Geometry check sheet. Reference: drawing and pictorial views, mm from the part's lowest x, y, z. A direction names the side the tool comes from. Give positions to 0.01 mm unless a question says otherwise; leave off trailing zeros. Order: outer loops, then holes, each group sorted by start corner. A loop starts at its lowest first (then second) coordinate and runs counter-clockwise, first axis right, second up. Notation, with made-up numbers: M 64.25,79.5 L 82.25,79.5 A19 cw 82.25,101.5 Z; hole C 57.5,-24 d1. An arc over 180 degrees is marked long. Use CSV: the item, a comma, the result in double quotes. Start each with the question number.
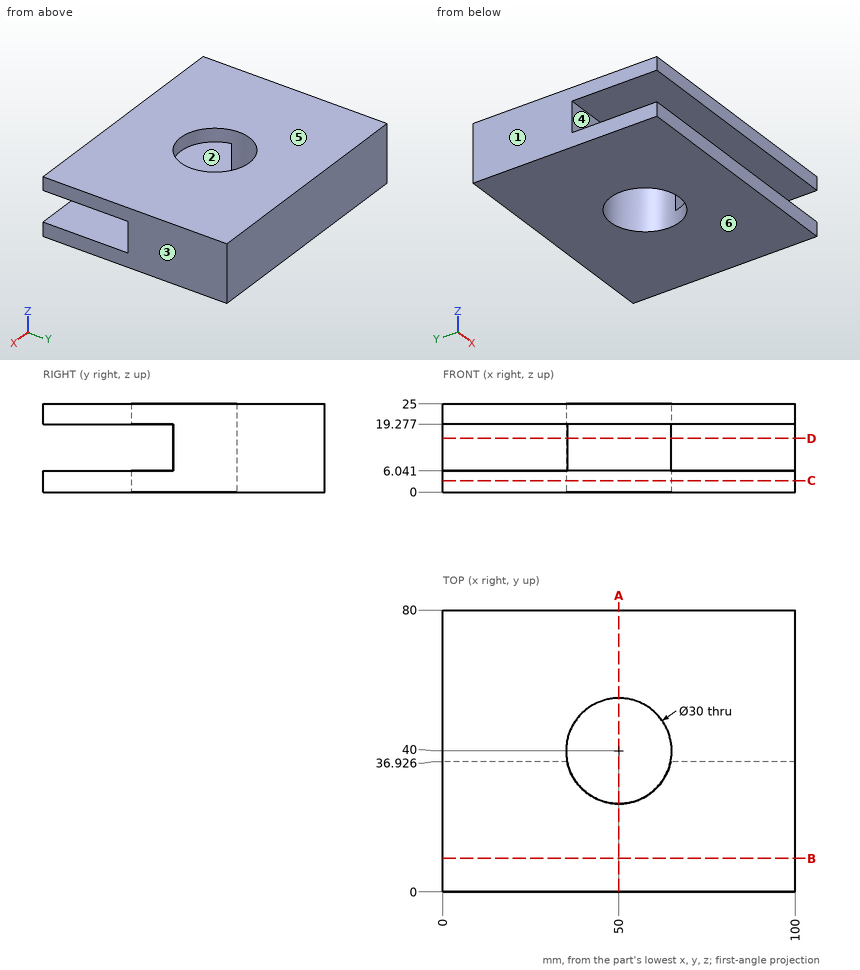
(1) Sectioned sample at A-A on x = 50. Record the cut outline in (y, z).
(2) Draft check along Z on the marked faces 3, 4, 5 and 6. Enter one of: +Z half, -Z half, draft (parallel to the pull), parting line (faces both ways), or undercut.
(3) Thickness scan on line 1 (Z direction, x = 17.5, y = 9); line 2 (Y direction, x = 50, z = 18.5); line 3 (Y direction, x = 50, z = 5.25). Record the ranges inside material, lowest first.
(4) Go/stop test with flat-tipped pins: P1, Ø18.5, axis at x = 34.5, y = 21.5, coming from the -Z side; P2, Ø6.5, axis at x = 15.5, z = 11, coming from the -Y side. Record where each tip stops, or that it passes through.
(5) Access from +Z, -Z, +X, -X, +Y, -Y to the whole of each face (thin tool, end or side, straight path). Record for the marked faces 1 and 2.
(6) Sectioned sample at B-B on y = 9.5. Record the cut outline in (x, z).
(7) Sectioned sample at C-C on z = 3.25. Record the cut outline in (x, y).
(8) Sectioned sample at D-D on z = 15.25. Record the cut outline in (x, y), then the cut area to 3 significant figures.
Responses:
1,outline,"M 0,0 L 25,0 L 25,6.04 L 0,6.04 Z; M 0,19.28 L 25,19.28 L 25,25 L 0,25 Z; M 55,0 L 80,0 L 80,25 L 55,25 Z"
2,face 3,"draft"
2,face 4,"undercut"
2,face 5,"+Z half"
2,face 6,"-Z half"
3,line 1,"0 to 6.04, 19.28 to 25"
3,line 2,"55 to 80"
3,line 3,"0 to 25, 55 to 80"
4,P1,"z = 0"
4,P2,"y = 36.93"
5,face 1,"+Z, -Z, -X, +Y, -Y"
5,face 2,"+X, -X, -Y"
6,outline,"M 0,0 L 100,0 L 100,6.04 L 0,6.04 Z; M 0,19.28 L 100,19.28 L 100,25 L 0,25 Z"
7,outline,"M 0,0 L 100,0 L 100,80 L 0,80 Z; hole C 50,40 d30"
8,outline,"M 0,36.93 L 35.32,36.93 A15 cw long 64.68,36.93 L 100,36.93 L 100,80 L 0,80 Z"
8,area,"3,860 mm2"
